The listing builds one solid part. Answer for the finished solid, in the listing's coordinates (mm). A direction names the side the tool comes from. Round coordinates to 2 decimals unless told otherwise and drop trailing zeros. Order: outer loops, then holes, each group sorted by start corner. A loop starts at its lowest first (then second) coordinate and runs counter-clockwise, first axis right, second up. Notation, with made-up numbers: M -27,41 L -15,41 A24 ccw -15,80 Z; hole C 38.25,43 d4. An arc over 180 degrees is marked long. Put each result on its own line as item: value. Start each with the question number.
1. The mould has two halves that part along Z. Classify faces 5 (the face through (-100, 13, 1)), 6 (the face through (60, -1, -1)), 7 (the face through (-1, 12, 61)): +Z half, -Z half, draft (parallel to the pull), parting line (faces both ways), or undercut.
2. Consider line 1 (X direction, y = 2.1, z = -40); line 2 (Z direction, x = -19, y = 7.25); line 3 (X direction, y = 10.5, z = 7.5). Determine where each line is inside the solid, lowest interval first.
3. The part is cut by section C-C (z = -40). Give the vertices of the cut face in (x, y).
4. The part is cut by section B-B (y = 8.75). Give the vertices of the cut face in (x, z), then the cut area to 3 significant figures.
5. Which of the six approach directions +Z, -Z, +X, -X, +Y, -Y give full straight-line access (tool end or side, diameter ignored) to faces 1 (the face through (25, -5, 22.5)), 2 (the face through (20, -4, -20)), 3 (the face through (-30, -4, -31)), 4 (the face through (-25, -4, -20))?
6. The part is cut by section D-D (x = -4). Give the vertices of the cut face in (y, z).
7. The part is cut by section A-A (x = 80). Give the vertices of the cut face in (y, z).
8. Each of these flat-tipped pins is pushed along its axis until it touches: pin 1 Ø1 at (y, z) = (-3, -19) entering from -X; pin 2 Ø3 at (x, z) = (72, 20.5) entering from -Y; pin 3 Ø4 at (x, y) = (23, -3.5) entering from +Z; pin 4 Ø8 at (y, z) = (-0.5, 30.5) entering from +X. Where does it stop, or does it pass through?
from build123d import *

# Parameters (mm, degrees)
SKETCH1_W             = 200
SKETCH1_H             = 120
BOSS_EXTRUDE3_DEPTH   = 3
SKETCH7_W             = 25
SKETCH7_H             = 120
BOSS_EXTRUDE4_DEPTH   = 1
SKETCH8_W             = 10
SKETCH8_H             = 5
BOSS_EXTRUDE5_DEPTH   = 2
BOSS_EXTRUDE5_2_DEPTH = 2
BOSS_EXTRUDE5_3_DEPTH = 2
BOSS_EXTRUDE5_4_DEPTH = 2
SKETCH10_W            = 10
SKETCH10_H            = 5
BOSS_EXTRUDE6_DEPTH   = 5
SKETCH11_R            = 5
CUT_EXTRUDE4_DEPTH    = 5
SKETCH13_W            = 6
SKETCH13_H            = 2
CUT_EXTRUDE5_DEPTH    = 130.77769454
FILLET3_R             = 1
FILLET4_R             = 1
SKETCH15_W            = 10
SKETCH15_H            = 5
BOSS_EXTRUDE9_DEPTH   = 7
SKETCH16_W            = 6
SKETCH16_H            = 2
CUT_EXTRUDE8_DEPTH    = 138.081180328
FILLET5_R             = 1
SKETCH18_W            = 120
SKETCH18_H            = 23
BOSS_EXTRUDE10_DEPTH  = 1
SKETCH19_W            = 202
SKETCH19_H            = 23
BOSS_EXTRUDE11_DEPTH  = 1
MIRROR2_START         = -62
MIRROR2_OUTLINE_W     = 202
MIRROR2_OUTLINE_H     = 23
MIRROR2_DEPTH         = 1
MIRROR2_START_2       = 60
MIRROR2_2_OUTLINE_W   = 202
MIRROR2_2_OUTLINE_H   = 23
MIRROR2_2_DEPTH       = 1


# Read off the part's stored shape, not the designer's step: Mirror2
with BuildPart() as part:
    # Sketch1 → Boss-Extrude3 (new body)
    with BuildSketch(Plane(origin=(0, 0, 0), x_dir=(1, 0, 0), z_dir=(0, 1, 0))):
        Rectangle(SKETCH1_W, SKETCH1_H)
    extrude(amount=BOSS_EXTRUDE3_DEPTH)

    # Sketch7 → Boss-Extrude4 (add)
    with BuildSketch(Plane(origin=(0, 0, 0), x_dir=(-1, 0, 0), z_dir=(0, -1, 0))):
        Rectangle(SKETCH7_W, SKETCH7_H)
        with Locations((60, 0)):
            Rectangle(SKETCH7_W, SKETCH7_H)
        with Locations((-60, 0)):
            Rectangle(SKETCH7_W, SKETCH7_H)
    extrude(amount=BOSS_EXTRUDE4_DEPTH)



with BuildPart() as body_2:
    # Sketch8 → Boss-Extrude5 (new body)
    with BuildSketch(Plane(origin=(0, -1, 0), x_dir=(-1, 0, 0), z_dir=(0, -1, 0))):
        with Locations((25, -20)):
            Rectangle(SKETCH8_W, SKETCH8_H)
    extrude(amount=-BOSS_EXTRUDE5_DEPTH)


with BuildPart() as body_3:
    # Sketch8 → Boss-Extrude5 2 (new body)
    with BuildSketch(Plane(origin=(0, -1, 0), x_dir=(-1, 0, 0), z_dir=(0, -1, 0))):
        with Locations((-25, -20)):
            Rectangle(SKETCH8_W, SKETCH8_H)
    extrude(amount=-BOSS_EXTRUDE5_2_DEPTH)


with BuildPart() as body_4:
    # Sketch8 → Boss-Extrude5 3 (new body)
    with BuildSketch(Plane(origin=(0, -1, 0), x_dir=(-1, 0, 0), z_dir=(0, -1, 0))):
        with Locations((-25, 20)):
            Rectangle(SKETCH8_W, SKETCH8_H)
    extrude(amount=-BOSS_EXTRUDE5_3_DEPTH)


with BuildPart() as body_5:
    # Sketch8 → Boss-Extrude5 4 (new body)
    with BuildSketch(Plane(origin=(0, -1, 0), x_dir=(-1, 0, 0), z_dir=(0, -1, 0))):
        with Locations((25, 20)):
            Rectangle(SKETCH8_W, SKETCH8_H)
    extrude(amount=-BOSS_EXTRUDE5_4_DEPTH)


with BuildPart() as part_1:
    add(part.part)

    add(body_2.part)  # Boss-Extrude6 merges body 2

    add(body_3.part)  # Boss-Extrude6 merges body 3

    add(body_4.part)  # Boss-Extrude6 merges body 4

    add(body_5.part)  # Boss-Extrude6 merges body 5
    # Sketch10 → Boss-Extrude6 (add)
    with BuildSketch(Plane(origin=(0, -1, 0), x_dir=(-1, 0, 0), z_dir=(0, -1, 0))):
        with Locations((25, -20)):
            Rectangle(SKETCH10_W, SKETCH10_H)
        with Locations((25, 20)):
            Rectangle(SKETCH10_W, SKETCH10_H)
        with Locations((-25, 20)):
            Rectangle(SKETCH10_W, SKETCH10_H)
        with Locations((-25, -20)):
            Rectangle(SKETCH10_W, SKETCH10_H)
    extrude(amount=BOSS_EXTRUDE6_DEPTH)

    # Sketch11 → Cut-Extrude4 (cut)
    with BuildSketch(Plane(origin=(0, 0, 0), x_dir=(-1, 0, 0), z_dir=(0, -1, 0))):
        with Locations(Location((-80, -40, 0), (0, 0, 90))):
            Circle(SKETCH11_R)
        with Locations(Location((-80, 40, 0), (0, 0, 90))):
            Circle(SKETCH11_R)
        with Locations(Location((80, 40, 0), (0, 0, 90))):
            Circle(SKETCH11_R)
        with Locations(Location((80, -40, 0), (0, 0, 90))):
            Circle(SKETCH11_R)
    extrude(amount=-CUT_EXTRUDE4_DEPTH, mode=Mode.SUBTRACT)

    # Sketch13 → Cut-Extrude5 (cut, through all)
    with BuildSketch(Plane(origin=(0, 0, -22.5), x_dir=(-1, 0, 0), z_dir=(0, 0, -1))):
        with Locations((25, -3)):
            Rectangle(SKETCH13_W, SKETCH13_H)
        with Locations((-25, -3)):
            Rectangle(SKETCH13_W, SKETCH13_H)
    extrude(amount=-CUT_EXTRUDE5_DEPTH, mode=Mode.SUBTRACT)

    # Fillet3
    fillet3_edges = [part_1.edges().sort_by_distance(p)[0] for p in [
        (30, 0, -20),
        (25, 0, -17.5),
        (20, 0, -20),
        (25, 0, -22.5),
    ]]
    fillet(fillet3_edges, radius=FILLET3_R)

    # Fillet4
    fillet4_edges = [part_1.edges().sort_by_distance(p)[0] for p in [
        (-25, 0, -22.5),
        (-20, 0, -20),
        (-25, 0, -17.5),
        (-30, 0, -20),
        (-25, 0, 22.5),
        (-30, 0, 20),
        (-25, 0, 17.5),
        (-20, 0, 20),
        (25, 0, 22.5),
        (20, 0, 20),
        (25, 0, 17.5),
        (30, 0, 20),
    ]]
    fillet(fillet4_edges, radius=FILLET4_R)

    # Sketch15 → Boss-Extrude9 (add)
    with BuildSketch(Plane(origin=(0, 0, 0), x_dir=(-1, 0, 0), z_dir=(0, -1, 0))):
        with Locations((-25, 31)):
            Rectangle(SKETCH15_W, SKETCH15_H)
        with Locations((25, 31)):
            Rectangle(SKETCH15_W, SKETCH15_H)
        with Locations((25, -31)):
            Rectangle(SKETCH15_W, SKETCH15_H)
        with Locations((-25, -31)):
            Rectangle(SKETCH15_W, SKETCH15_H)
    extrude(amount=BOSS_EXTRUDE9_DEPTH)

    # Sketch16 → Cut-Extrude8 (cut, through all)
    with BuildSketch(Plane.XY.offset(33.5)):
        with Locations((25, -3)):
            Rectangle(SKETCH16_W, SKETCH16_H)
        with Locations((-25, -3)):
            Rectangle(SKETCH16_W, SKETCH16_H)
    extrude(amount=-CUT_EXTRUDE8_DEPTH, mode=Mode.SUBTRACT)

    # Fillet5
    fillet5_edges = [part_1.edges().sort_by_distance(p)[0] for p in [
        (30, 0, -31),
        (25, 0, -28.5),
        (20, 0, -31),
        (25, 0, -33.5),
        (-20, 0, -31),
        (-25, 0, -28.5),
        (-30, 0, -31),
        (-25, 0, -33.5),
        (-25, 0, 28.5),
        (-20, 0, 31),
        (-25, 0, 33.5),
        (-30, 0, 31),
        (20, 0, 31),
        (25, 0, 28.5),
        (30, 0, 31),
        (25, 0, 33.5),
    ]]
    fillet(fillet5_edges, radius=FILLET5_R)

    # Sketch18 → Boss-Extrude10 (add)
    with BuildSketch(Plane(origin=(100, 0, 0), x_dir=(0, 0, -1), z_dir=(1, 0, 0))):
        with Locations((0, 11.5)):
            Rectangle(SKETCH18_W, SKETCH18_H)
    boss_extrude10 = extrude(amount=BOSS_EXTRUDE10_DEPTH)

    # Mirror1: Boss-Extrude10 across plane
    add(boss_extrude10.mirror(Plane(origin=(0, 0, 0), x_dir=(0, 0, 1), z_dir=(1, 0, 0))))

    # Sketch19 → Boss-Extrude11 (add)
    with BuildSketch(Plane(origin=(0, 0, -60), x_dir=(-1, 0, 0), z_dir=(0, 0, -1))):
        with Locations((0, 11.5)):
            Rectangle(SKETCH19_W, SKETCH19_H)
    extrude(amount=BOSS_EXTRUDE11_DEPTH)

    # Mirror2 outline → Mirror2 (add)
    with BuildSketch(Plane.XY.offset(MIRROR2_START)):
        with Locations((0, 11.5)):
            Rectangle(MIRROR2_OUTLINE_W, MIRROR2_OUTLINE_H)
    extrude(amount=MIRROR2_DEPTH)

    # Mirror2 2 outline → Mirror2 2 (add)
    with BuildSketch(Plane.XY.offset(MIRROR2_START_2)):
        with Locations((0, 11.5)):
            Rectangle(MIRROR2_2_OUTLINE_W, MIRROR2_2_OUTLINE_H)
    extrude(amount=MIRROR2_2_DEPTH)


solid = part_1.part
Resolved:
1. face 5: undercut
1. face 6: draft
1. face 7: +Z half
2. line 1: -101 to -85, -75 to 75, 85 to 101
2. line 2: -62 to -60, 60 to 61
2. line 3: -101 to -100, 100 to 101
3. outline: M -101,0 L -85,0 L -85,3 L -100,3 L -100,23 L -101,23 Z; M -75,0 L -72.5,0 L -72.5,-1 L -47.5,-1 L -47.5,0 L -12.5,0 L -12.5,-1 L 12.5,-1 L 12.5,0 L 47.5,0 L 47.5,-1 L 72.5,-1 L 72.5,0 L 75,0 L 75,3 L -75,3 Z; M 85,0 L 101,0 L 101,23 L 100,23 L 100,3 L 85,3 Z
4. outline: M -101,-62 L 101,-62 L 101,61 L -101,61 Z; hole M -100,-60 L 100,-60 L 100,60 L -100,60 Z
4. area: 846 mm2
5. face 1: +X, -X, -Y
5. face 2: +Z, -Z, -Y
5. face 3: +Z, -Z, -X, -Y
5. face 4: +Z, -Z
6. outline: M -1,-60 L 0,-60 L 0,-62 L 23,-62 L 23,-60 L 3,-60 L 3,60 L 23,60 L 23,61 L 0,61 L 0,60 L -1,60 Z
7. outline: M 0,-62 L 23,-62 L 23,-60 L 3,-60 L 3,-45 L 0,-45 Z; M 0,-35 L 3,-35 L 3,35 L 0,35 Z; M 0,45 L 3,45 L 3,60 L 23,60 L 23,61 L 0,61 Z
8. pin 1: x = -30
8. pin 2: y = -1
8. pin 3: z = 33.5
8. pin 4: x = 101
